Design review of the part shown in the three views and the two pictorial views. Dimensions are in mm from the part's minimum x, y and z. A direction names the side the tool comes from. Give positions to 0.01 mm unless a question says otherwise; leave off trailing zeros. Order: outer loops, then holes, each group sorted by start corner. A loop starts at its lowest first (then second) coordinate and runs counter-clockwise, first axis right, second up.
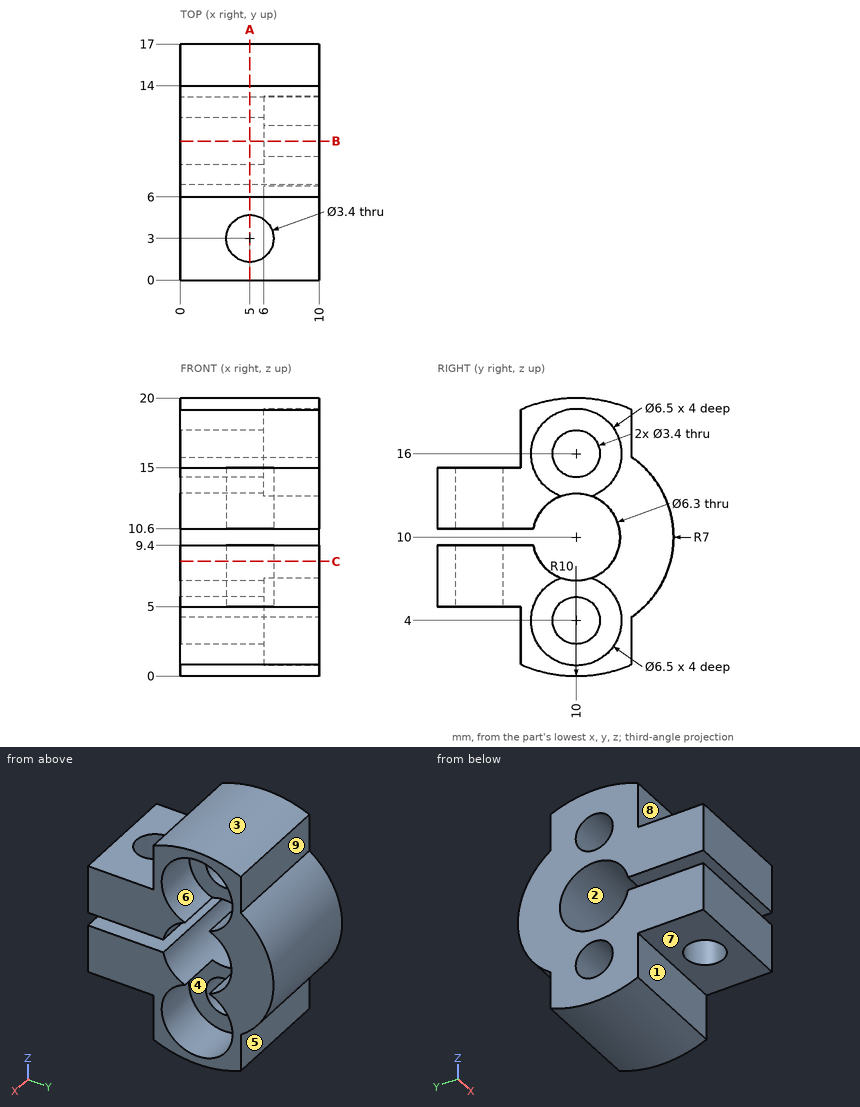
Item 1: Take a section at A-A (x = 5). Give the number of separate pieces and of enclosed holes in the cut face, and give its area (3 significant figures).
Values found:
separate pieces: 3
enclosed holes: 2
area: 152 mm2
Item 2: Draft analysis for pull direction Z (two halves, no side actions). For the marked faces 1, 2, 3 and 4, state which applies: released by +Z, released by -Z, zero draft, split by the parting line, or undercut.
Values found:
face 1: zero draft
face 2: undercut
face 3: released by +Z
face 4: undercut
Item 3: For line 1 (Z direction, x = 2.75, y = 2); line 2 (Y direction, x = 6.75, z = 16); line 3 (Z direction, x = 5, y = 9.75), list the stretches that pass through material, from the lowest coordinate up.
Values found:
line 1: z = 5 to 9.4, 10.6 to 15
line 2: y = 6 to 6.75, 13.25 to 14
line 3: z = 0 to 2.32, 5.68 to 6.86, 13.14 to 14.32, 17.68 to 20
Item 4: Take a section at B-B (y = 10). Give the boundary of the cut face in (x, z).
Values found:
outline: (0, 0) - (10, 0) - (10, 0.75) - (6, 0.75) - (6, 2.3) - (0, 2.3) - close; (0, 5.7) - (6, 5.7) - (6, 6.85) - (0, 6.85) - close; (0, 13.15) - (6, 13.15) - (6, 14.3) - (0, 14.3) - close; (0, 17.7) - (6, 17.7) - (6, 19.25) - (10, 19.25) - (10, 20) - (0, 20) - close
Item 5: Take a section at C-C (z = 8.25). Give the boundary of the cut face in (x, y).
Values found:
outline: (0, 0) - (10, 0) - (10, 7.38) - (0, 7.38) - close; (0, 12.62) - (10, 12.62) - (10, 16.78) - (0, 16.78) - close; hole circle Ø3.4 at (5, 3)
Item 6: Clearance check with flat-ended pins moving along their axes: pin 1 Ø5 at (y, z) = (10, 4) entering from +X; pin 2 Ø1.7 at (x, z) = (7, 2) entering from +Y; pin 3 Ø3 at (x, y) = (7, 8) entering from +Z. State where each tip first meets the part, or that it passes through.
Values found:
pin 1: stops at x = 6
pin 2: stops at y = 14
pin 3: stops at z = 19.99
Item 7: For the marked faces 5, 6, 7, 8 and 9, list the 3-axis set-ups (+Z, -Z, +X, -X, +Y, -Y) from which the entire face can be reached by the end or side of a thin tool; tool diameter is ignored.
Values found:
face 5: -Z, +X, -X, +Y
face 6: +X
face 7: -Z, +X, -X, -Y
face 8: +Z, +X, -X, -Y
face 9: +Z, +X, -X, +Y
